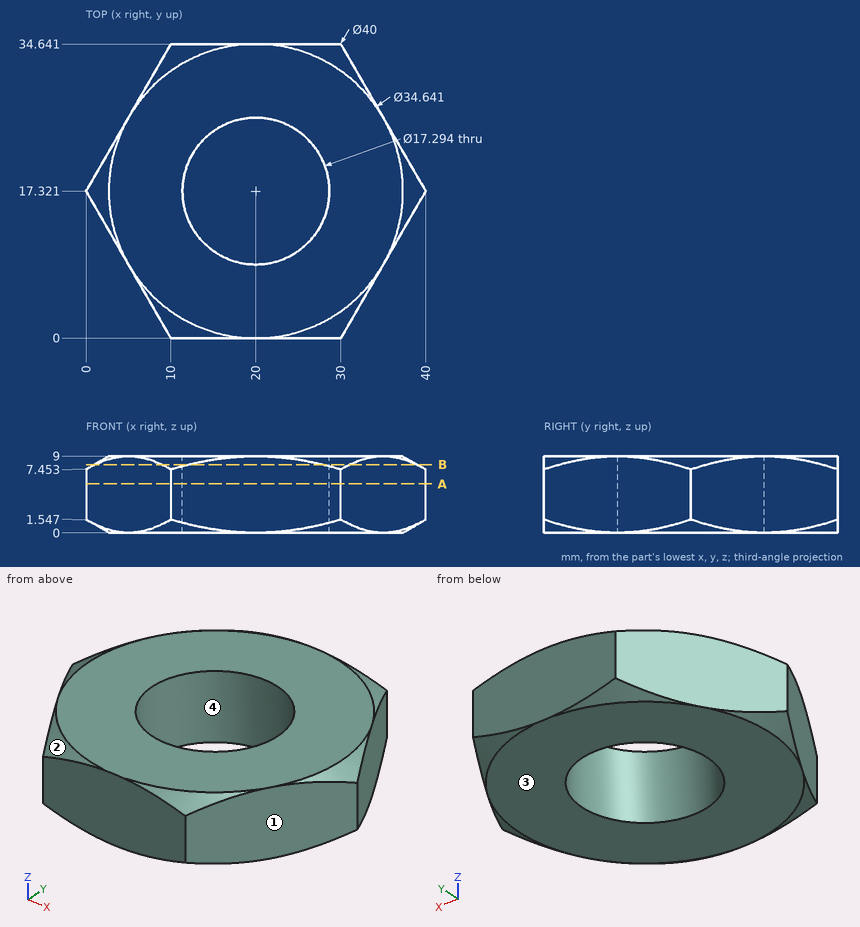
Geometry check sheet. Reference: drawing and pictorial views, mm from the part's lowest x, y, z. Give positions to 0.01 mm unless a question says otherwise; leave off trailing zeros. Order: outer loops, then holes, each group sorted by start corner. A loop starts at its lowest first (then second) coordinate and runs counter-clockwise, first axis right, second up. Notation, with made-up numbers: M 43.5,45 L 91.5,45 A16 cw 91.5,69 Z; hole C -18,47 d5. An arc over 180 degrees is marked long. Answer in a Markdown table with one row per item.
1) Gauge pin test, flat ends, axial feed: P1, Ø1, axis at y = 16.5, z = 4.5, coming from the -X side (1 decimal); P2, Ø5, axis at y = 8.5, z = 3.5, coming from the +X side. Record the tip position at first contact, or that the pin passes through.
Filled sheet:
| item | result |
|---|---|
| P1 | stops at x = 0.2 |
| P2 | stops at x = 36.35 |
2) Release check for a two-part mould opening along Y. For the marked faces 1, 2, 3 and 4 record: +Y half, -Y half, draft (parallel to the pull), parting line (faces both ways), or undercut.
Filled sheet:
| item | result |
|---|---|
| face 1 | -Y half |
| face 2 | parting line |
| face 3 | draft |
| face 4 | undercut |
3) Cross-section at B-B, the plane z = 8. Enter the section's corners in (x, y) (1 decimal).
Filled sheet:
| item | result |
|---|---|
| outline | M 1,15.5 L 9,1.8 A19.1 ccw 12.1,0 L 27.9,0 A19.1 ccw 31,1.8 L 39,15.5 A19.1 ccw 39,19.1 L 31,32.9 A19.1 ccw 27.9,34.6 L 12.1,34.6 A19.1 ccw 9,32.9 L 1,19.1 A19.1 ccw Z; hole C 20,17.3 d17.3 |
4) Cross-section at A-A, the plane z = 5.75. Enter the section's corners in (x, y) (1 decimal).
Filled sheet:
| item | result |
|---|---|
| outline | M 0,17.3 L 10,0 L 30,0 L 40,17.3 L 30,34.6 L 10,34.6 Z; hole C 20,17.3 d17.3 |
5) Thickness scan on L1, parallel to X at y = 14.5, z = 1.5 (1 decimal); L2, parallel to X at y = 25, z = 8 (1 decimal); L3, parallel to Z at x = 8.5, y = 30.5. Record the ranges inside material, lowest first. Write a range as [from, to].
Filled sheet:
| item | result |
|---|---|
| L1 | x = [1.6, 11.8], [28.2, 38.4] |
| L2 | x = [4.4, 16], [24, 35.6] |
| L3 | z = [0.1, 8.9] |
